Geometry: final body of the model. Coordinates: model frame, mm. A direction names the side the tool comes from. Give positions to 0.01 mm unless a question says otherwise; leave off trailing zeros. Order: outer loops, then holes, each group sorted by start corner. A loop starts at its lowest first (then second) coordinate and runs counter-clockwise, first axis right, second up. Notation, with made-up numbers: M 81.25,22.25 L 117.25,22.25 A9 cw 117.25,29.25 Z; hole C 31.25,88 d10. An arc over 180 degrees is marked long. One line per item, written item: value. Start each with the question number.
Autodesk Inventor part; units mm, degrees
ref_plane "YZ Plane" through (0, 0, 0) normal (1, 0, 0) x (0, 1, 0)
ref_plane "XZ Plane" through (0, 0, 0) normal (0, 1, 0) x (-1, 0, 0)
ref_plane "XY Plane" through (0, 0, 0) normal (0, 0, 1) x (1, 0, 0)
sketch "Sketch1" plane through (0, 0, 0) normal (0, 0, 1) x (1, 0, 0)
  line L0 (0, 0) -> (11.3, 0)
  line L1 (11.3, 0) -> (11.3, 11.2)
  line L2 (11.3, 11.2) -> (10.2, 11.2)
  line L3 (10.2, 11.2) -> (10.2, 1.1)
  line L4 (10.2, 1.1) -> (1.1, 1.1)
  line L5 (1.1, 1.1) -> (1.1, 11.2)
  line L6 (1.1, 11.2) -> (0, 11.2)
  line L7 (0, 11.2) -> (0, 0)
  dimension "d0" = 1.1
  dimension "d1" = 1.1
  dimension "d2" = 11.3
  dimension "d3" = 11.2
extrude "Extrusion1" add sketch "Sketch1" along normal blind 7.4
fillet "Fillet1" radius 3.7 4 edges at (10.75, 11.2, 7.4) (10.75, 11.2, 0) (0.55, 11.2, 7.4) (0.55, 11.2, 0)
sketch "Sketch2" plane through (11.3, 0, 7.4) normal (1, 0, 0) x (0, 0, -1)
  line L0 (7.4, 0) -> (0, 0)
  point P0 (3.7, 7.5)
  dimension "d14" = 7.5
hole "Hole1" at (11.3, 7.5, 3.7) direction (-1, 0, 0) diameter 4.25 depth 14 tip angle 118
fillet "Fillet2" radius 1.1 4 edges at (1.1, 1.1, 3.7) (0, 0, 3.7) (11.3, 0, 3.7) (10.2, 1.1, 3.7)
sketch "Sketch3" plane through (2.2, 1.1, 0) normal (0, 1, 0) x (1, 0, 0)
  line L0 (6.9, 0) -> (0, 0)
  point P0 (-2.2, 0)
  point P1 (3.45, -3.7)
  point P2 (3.45, 0)
hole "Hole2" at (5.65, 1.1, 3.7) direction (0, -1, 0) diameter 4.25 depth 14 tip angle 118
properties part number "Linear Actuator Rear Mount"
Q1. Section query B-B on x = 5.65. Return loops of the section in (y, z) (3 decimals), and give its area (4 significant figures).
Q2. Set-up query: faces 1 (the face through (10.742, 10.145, 1.112)), 2 (the face through (9.869, 1.414, 3.752)). Return all of +Z, -Z, +X, -X, +Y, -Y with unobstructed straight access to the full face (end or side cutting, diameter ignored); none if empty.
Q3. Mould query, pull axis X, two halves, no side actions, for faces 3 (the face through (0.314, 0.331, 3.752)), 4 (the face through (10.969, 0.314, 3.752)), 5 (the face through (8, 0, 3)), 6 (the face through (1.1, 5, 4)). Classes: +X half, -X half, draft (parallel to the pull), parting line (faces both ways), or undercut.
Q4. Ray query, line 1 along Z through (x, y) = (5.65, 0.9) (3 decimals); line 2 along X through (y, z) = (5.5, 6); line 3 along Y through (x, z) = (8.5, 2.25). Return the intervals inside material, ascending. Write a range as [from, to].
Q5. Section query A-A on y = 4. Return loops of the section in (x, z), and give its area (3 significant figures).
Q6. Section query C-C on z = 2.25. Return loops of the section in (x, y).
Q7. Contact query for a flat-ended pin moving along its axis: pin 1 (3.5 mm diameter, centred on x = 5, z = 2, fed in from +Y). Output: stop coordinate, or through.
Q8. Section query D-D on x = 2.75. Return loops of the section in (y, z), and give its area (3 significant figures).
Results below:
1. outline: M 0,0 L 1.1,0 L 1.1,1.575 L 0,1.575 Z; M 0,5.825 L 1.1,5.825 L 1.1,7.4 L 0,7.4 Z
1. area: 3.465 mm2
2. face 1: -Z, +X, -X, +Y
2. face 2: +Z, -Z, +Y
3. face 3: -X half
3. face 4: +X half
3. face 5: draft
3. face 6: undercut
4. line 1: [0, 1.575], [5.825, 7.4]
4. line 2: [0, 1.1], [10.2, 11.3]
4. line 3: [0, 1.1]
5. outline: M 0,0 L 1.1,0 L 1.1,7.4 L 0,7.4 Z; M 10.2,0 L 11.3,0 L 11.3,7.4 L 10.2,7.4 Z
5. area: 16.3 mm2
6. outline: M 0,1.1 A1.1 ccw 1.1,0 L 4.1,0 L 4.1,1.1 L 2.2,1.1 A1.1 cw 1.1,2.2 L 1.1,5.95 L 0,5.95 Z; M 0,9.05 L 1.1,9.05 L 1.1,10.9 L 0,10.9 Z; M 7.2,0 L 10.2,0 A1.1 ccw 11.3,1.1 L 11.3,5.95 L 10.2,5.95 L 10.2,2.2 A1.1 cw 9.1,1.1 L 7.2,1.1 Z; M 10.2,9.05 L 11.3,9.05 L 11.3,10.9 L 10.2,10.9 Z
7. pin 1: y = 1.1
8. outline: M 0,0 L 1.1,0 L 1.1,7.4 L 0,7.4 Z
8. area: 8.14 mm2
